Geometry check sheet. Reference: drawing and pictorial views, mm from the part's lowest x, y, z. A direction names the side the tool comes from. Coordinates: 2 decimals unless noted, no trailing zeros. Write each loop counter-clockwise with the first axis right and the second up, starting at its lowest first coordinate (ties: lowest second). Pieces come first, ordered by that corner, then holes. Notation, with made-up numbers: (-28, -21) - (-1, -21) arc R26 cw to (-1, 16) - close; hole circle Ø1 at (17.5, 25.25). An arc over 180 degrees is marked (long way). Answer as CSV lines item,"result". Start each with the question number.
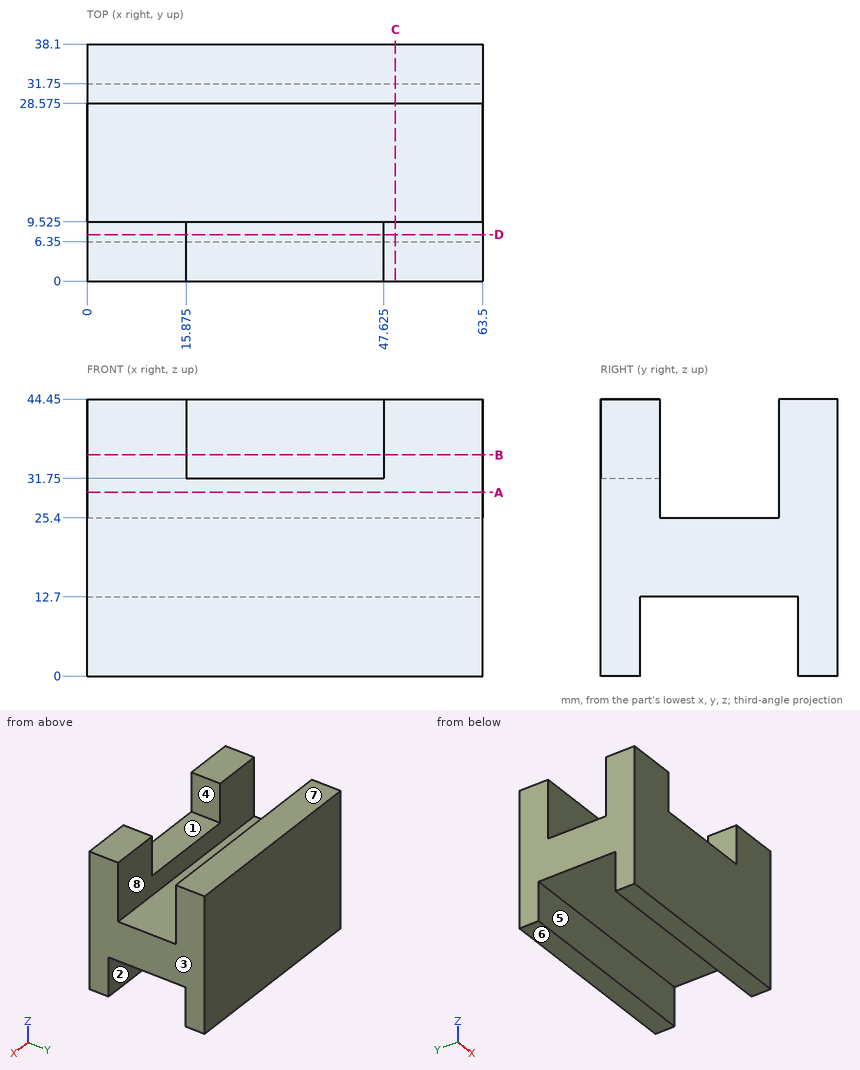
1. Cross-section at A-A (z = 29.5). Record the cut outline in (x, y) (3 decimals), and give its area (3 significant figures).
2. Scan lines: line 1 along X through (y, z) = (6, 34) (3 decimals); line 2 along Y through (x, z) = (5, 33.5) (3 decimals); line 3 along Y through (x, z) = (15, 4.5). Record each from-to range of solid material in increasing order. Write a range as from..to.
3. Cross-section at B-B (z = 35.5). Record the cut outline in (x, y) (3 decimals).
4. Access from +Z, -Z, +X, -X, +Y, -Y to the whole of each face (thin tool, end or side, straight path). Record for the marked faces 4, 5, 6, 7 and 8.
5. Cross-section at D-D (y = 7.5). Record the cut outline in (x, z) (3 decimals), and give its area (3 significant figures).
6. Cross-section at C-C (x = 49.5). Record the cut outline in (y, z) (3 decimals).
7. Depth check by flat-ended pin: P1, Ø12, axis at x = 24.5, y = 24.5, coming from the +Z side; P2, Ø3, axis at x = 12, y = 21, coming from the +Z side; P3, Ø20.5, axis at x = 43.5, y = 17, coming from the -Z side; P4, Ø10.5, axis at x = 24.5, y = 4.5, coming from the +Z side. Enter the tip coordinate at first touch or a pass-through.
8. Draft check along X on the marked faces 1, 2 and 3. Enter one of: pulls with the +X half, pulls with the -X half, needs draft (parallel to the pull), parting line crosses it, or undercut.
Completed:
1,outline,"(0, 0) - (63.5, 0) - (63.5, 9.525) - (0, 9.525) - close; (0, 28.575) - (63.5, 28.575) - (63.5, 38.1) - (0, 38.1) - close"
1,area,"1,210 mm2"
2,line 1,"x = 0..15.875, 47.625..63.5"
2,line 2,"y = 0..9.525, 28.575..38.1"
2,line 3,"y = 0..6.35, 31.75..38.1"
3,outline,"(0, 0) - (15.875, 0) - (15.875, 9.525) - (0, 9.525) - close; (0, 28.575) - (63.5, 28.575) - (63.5, 38.1) - (0, 38.1) - close; (47.625, 0) - (63.5, 0) - (63.5, 9.525) - (47.625, 9.525) - close"
4,face 4,"+Z, -Y"
4,face 5,"-Z, +X, -X"
4,face 6,"-Z, +X, -X, +Y, -Y"
4,face 7,"+Z, +X, -X, +Y, -Y"
4,face 8,"+Z, +X, -X"
5,outline,"(0, 12.7) - (63.5, 12.7) - (63.5, 44.45) - (47.625, 44.45) - (47.625, 31.75) - (15.875, 31.75) - (15.875, 44.45) - (0, 44.45) - close"
5,area,"1,610 mm2"
6,outline,"(0, 0) - (6.35, 0) - (6.35, 12.7) - (31.75, 12.7) - (31.75, 0) - (38.1, 0) - (38.1, 44.45) - (28.575, 44.45) - (28.575, 25.4) - (9.525, 25.4) - (9.525, 44.45) - (0, 44.45) - close"
7,P1,"stops at z = 44.45"
7,P2,"stops at z = 25.4"
7,P3,"stops at z = 12.7"
7,P4,"stops at z = 31.75"
8,face 1,"undercut"
8,face 2,"needs draft"
8,face 3,"pulls with the +X half"
